from build123d import *

# Parameters (mm, degrees)
BOSS_EXTRUDE2_DEPTH     = 6
SKETCH3_R               = 5.196152423
SKETCH3_R_2             = 2.5
BOSS_EXTRUDE4_DEPTH     = 12
CUT_EXTRUDE2_REACH      = 21.672
SKETCH1_4_R             = 2
CUT_EXTRUDE3_REACH      = 23.633
CUT_EXTRUDE3_END_RADIUS = 2.5
SKETCH4_R               = 1.5
FILLET3_R               = 0.3


with BuildPart() as part:
    # Sketch1 → Boss-Extrude2 (new body)
    with BuildSketch(Plane(origin=(0, 0, 0), x_dir=(1, 0, 0), z_dir=(0, 1, 0))):
        Polygon((-3, 5.196152423), (-6, 0), (-3, -5.196152423), (3, -5.196152423), (6, 0), (3, 5.196152423), align=None)
    extrude(amount=BOSS_EXTRUDE2_DEPTH)

    # Sketch3 → Boss-Extrude4 (add)
    with BuildSketch(Plane(origin=(0, 6, 0), x_dir=(1, 0, 0), z_dir=(0, 1, 0))):
        with Locations(Location((0, 0, 0), (0, 0, 270))):
            Circle(SKETCH3_R)
        with Locations(Location((0, 0, 0), (0, 0, 270))):
            Circle(SKETCH3_R_2, mode=Mode.SUBTRACT)
    extrude(amount=BOSS_EXTRUDE4_DEPTH)

    # Sketch1<4> → Cut-Extrude2 (cut, up to next)
    with BuildSketch(Plane(origin=(0, 0, 0), x_dir=(1, 0, 0), z_dir=(0, 1, 0)), mode=Mode.PRIVATE) as cut_extrude2_sk1:
        with Locations(Location((0, 0, 0), (0, 0, 270))):
            Circle(SKETCH1_4_R)
    cut_extrude2_tool1 = extrude(cut_extrude2_sk1.sketch, amount=CUT_EXTRUDE2_REACH, mode=Mode.PRIVATE) & part.part
    add(cut_extrude2_tool1.solids().sort_by_distance((0, 0, 0))[0], mode=Mode.SUBTRACT)

    # Cut-Extrude3: up to this cylinder (the profile starts outside it)
    cut_extrude3_end = Plane(origin=(0, 13.714513, 0), z_dir=(0, -1, 0)) * Cylinder(CUT_EXTRUDE3_END_RADIUS, 53.266, mode=Mode.PRIVATE)
    # Sketch4 → Cut-Extrude3 (cut, up to the surface)
    with BuildSketch(Plane.XY.offset(5.196152423), mode=Mode.PRIVATE) as cut_extrude3_sk1:
        with Locations((0, 13.714512782)):
            Circle(SKETCH4_R)
    cut_extrude3_tool1 = extrude(cut_extrude3_sk1.sketch, amount=-CUT_EXTRUDE3_REACH, mode=Mode.PRIVATE) - cut_extrude3_end
    add(cut_extrude3_tool1.solids().sort_by_distance((0, 13.714513, 5.196152))[0], mode=Mode.SUBTRACT)

    # Fillet3
    fillet3_edges = [part.edges().sort_by_distance(p)[0] for p in [
        (0, 18, -5.196152423),
        (0, 18, -2.5),
        (0, 0, -2),
        (-1.5, 13.714512782, 4.974937186),
    ]]
    fillet(fillet3_edges, radius=FILLET3_R)


solid = part.part
Can you work these out from the model? Positions are in its coordinate system, mm. A direction names the side the tool comes from. Coordinates: 2 decimals unless noted, no trailing zeros. Write each loop counter-clockwise with the first axis right and the second up, starting at its lowest first coordinate (ties: lowest second). Pieces come first, ordered by that corner, then holes. Notation, with made-up numbers: (79.5, -28) - (124.5, -28) arc R24 ccw to (124.5, 0) - close; hole circle Ø6 at (43, 30.5). An arc over 180 degrees is marked (long way). Return JSON: item names as keys, results as strings. Group by question number.
Item 1: I'm going to push flat-ended pins straight in: pin 1 Ø1.5 at (y, z) = (13, -3.5) entering from +X; pin 2 Ø3 at (x, y) = (2, 10.5) entering from -Z; pin 3 Ø2 at (y, z) = (16, 4) entering from +X. Where does each tip first touch, or does it pass through?
Item 2: Which directions (+Z, -Z, +X, -X, +Y, -Y) give clear straight access to the entire face, cutting with the end or side of a thin tool? Please do faces 4 (the face through (-2.6, 6, -4.7)), 5 (the face through (2.7, 6, 4.7)), 6 (the face through (0.1, 11.8, -2.5)), 7 (the face through (-2.6, 6, 4.7)), 8 (the face through (1.386, 13.14, 3.468)).
Item 3: We'd pull the mould along Z, two halves only. Please class faces 1 (the face through (0, 3, -5.196)), 2 (the face through (5.4, 6, 0)), 3 (the face through (-2, 3, 0)): pulls with the +Z half, pulls with the -Z half, needs draft (parallel to the pull), parting line crosses it, or undercut.
Item 4: Please list where these lines run through material, in increasing order: probe 1 along Z at (x, y) = (4.5, 10.75); probe 2 along Z at (x, y) = (-1.5, 17).
Item 5: If we section it at A-A (y = 9.5): Write out the boundary of the cut face in (x, z), then the cut area to 3 significant figures.
Return value:
{
 "1": {"pin 1": "stops at x = 4.41", "pin 2": "stops at z = -5.17", "pin 3": "stops at x = 4.24"},
 "2": {"face 4": "-Z, -X, +Y", "face 5": "+Z, +X, +Y", "face 6": "+Y", "face 7": "+Z, -X, +Y", "face 8": "+Z"},
 "3": {"face 1": "pulls with the -Z half", "face 2": "needs draft", "face 3": "undercut"},
 "4": {"probe 1": "z = -2.6 to 2.6", "probe 2": "z = -4.97 to -2, 2 to 4.97"},
 "5": {"outline": "circle Ø10.39 at (0, 0); hole circle Ø5 at (0, 0)", "area": "65.2 mm^2"}
}
